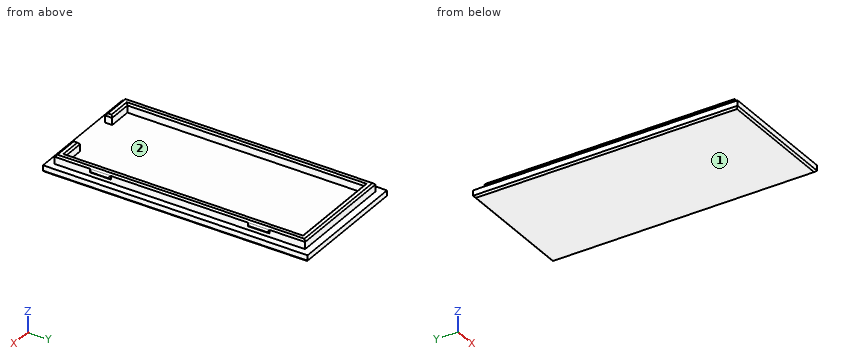
```python
from build123d import *

# Parameters (mm, degrees)
F1_W     = 2
F1_H     = 6.165323171
F1_H_2   = 5.8635988384
F1_H_3   = 38.7710779905
F1_W_2   = 14
F1_H_4   = 2
F1_W_3   = 26.8
F1_H_5   = 8
F1_W_4   = 0.5
F2_DEPTH = 2
F3_START = 1
F3_DEPTH = 3.5
F4_START = 3
F4_DEPTH = 1
F5_SIZE  = 0.49999


# Not quite as in the source:
# - a fillet or chamfer is up to 0.001 mm smaller than in the source, because OpenCascade refuses the exact size


with BuildPart() as f2:
    # F1 (on Top) → F2 (new body)
    with BuildSketch(Plane.XY):
        Polygon((16.0419130247, 37.7546238333), (-14.7580869753, 37.7546238333), (-14.7580869753, 27.7546238333), (-12.7580869753, 27.7546238333), (-12.7580869753, 35.7546238333), (14.0419130247, 35.7546238333), (14.0419130247, 27.7546238333), (16.0419130247, 27.7546238333), align=None)
        Polygon((-12.7580869753, -23.0453761667), (-14.7580869753, -23.0453761667), (-14.7580869753, -26.0453761667), (-14.7580869753, -33.0453761667), (-6.0801735182, -33.0453761667), (-6.0801735182, -31.0453761667), (-12.7580869753, -31.0453761667), align=None)
        with Locations((-13.7580869753, 24.6719622478)):
            Rectangle(F1_W, F1_H)
        with Locations((-13.7580869753, -20.1135767475)):
            Rectangle(F1_W, F1_H_2)
        Polygon((-12.7580869753, 21.5893006623), (-14.7580869753, 21.5893006623), (-14.7580869753, -3.2453761667), (-14.7580869753, -17.1817773283), (-12.7580869753, -17.1817773283), align=None)
        with Locations((15.0419130247, 2.203761667)):
            Rectangle(F1_W, F1_H_3)
        with Locations((15.0419130247, -20.1135767475)):
            Rectangle(F1_W, F1_H_2)
        Polygon((16.0419130247, -33.0453761667), (16.0419130247, -23.0453761667), (14.0419130247, -23.0453761667), (14.0419130247, -31.0453761667), (7.9198264818, -31.0453761667), (7.9198264818, -33.0453761667), align=None)
        with Locations((15.0419130247, 24.6719622478)):
            Rectangle(F1_W, F1_H)
        Polygon((-14.7580869753, -26.0453761667), (-16.7580869753, -26.0453761667), (-16.7580869753, -35.0453761667), (-6.0801735182, -35.0453761667), (-6.0801735182, -33.0453761667), (-14.7580869753, -33.0453761667), align=None)
        with Locations((0.9198264818, -32.0453761667)):
            Rectangle(F1_W_2, F1_H_4)
        with Locations((0.9198264818, -34.0453761667)):
            Rectangle(F1_W_2, F1_H_4)
        with Locations((0.6419130247, 24.6719622478)):
            Rectangle(F1_W_3, F1_H)
        with Locations((0.6419130247, 2.203761667)):
            Rectangle(F1_W_3, F1_H_3)
        Polygon((14.0419130247, -23.0453761667), (-12.7580869753, -23.0453761667), (-12.7580869753, -31.0453761667), (-6.0801735182, -31.0453761667), (7.9198264818, -31.0453761667), (14.0419130247, -31.0453761667), align=None)
        Polygon((-14.7580869753, 27.7546238333), (-14.7580869753, 37.7546238333), (16.0419130247, 37.7546238333), (16.0419130247, 27.7546238333), (16.5419130247, 27.7546238333), (16.5419130247, 21.5893006623), (16.0419130247, 21.5893006623), (16.0419130247, -17.1817773283), (16.5419130247, -17.1817773283), (16.5419130247, -23.0453761667), (16.0419130247, -23.0453761667), (16.0419130247, -33.0453761667), (7.9198264818, -33.0453761667), (7.9198264818, -35.0453761667), (18.0419130247, -35.0453761667), (18.0419130247, 39.7546238333), (-16.7580869753, 39.7546238333), (-16.7580869753, -3.2453761667), (-14.7580869753, -3.2453761667), (-14.7580869753, 21.5893006623), (-15.2580869753, 21.5893006623), (-15.2580869753, 27.7546238333), align=None)
        with Locations((0.6419130247, 31.7546238333)):
            Rectangle(F1_W_3, F1_H_5)
        Polygon((-14.7580869753, -17.1817773283), (-14.7580869753, -3.2453761667), (-16.7580869753, -3.2453761667), (-16.7580869753, -26.0453761667), (-14.7580869753, -26.0453761667), (-14.7580869753, -23.0453761667), (-15.2580869753, -23.0453761667), (-15.2580869753, -17.1817773283), align=None)
        with Locations((0.6419130247, -20.1135767475)):
            Rectangle(F1_W_3, F1_H_2)
        with Locations((-15.0080869753, -20.1135767475)):
            Rectangle(F1_W_4, F1_H_2)
        with Locations((-15.0080869753, 24.6719622478)):
            Rectangle(F1_W_4, F1_H)
        with Locations((16.2919130247, -20.1135767475)):
            Rectangle(F1_W_4, F1_H_2)
        with Locations((16.2919130247, 24.6719622478)):
            Rectangle(F1_W_4, F1_H)
    extrude(amount=F2_DEPTH)

    # F1 (on Top) → F3 (join)
    with BuildSketch(Plane.XY.offset(F3_START)):
        Polygon((16.0419130247, 37.7546238333), (-14.7580869753, 37.7546238333), (-14.7580869753, 27.7546238333), (-12.7580869753, 27.7546238333), (-12.7580869753, 35.7546238333), (14.0419130247, 35.7546238333), (14.0419130247, 27.7546238333), (16.0419130247, 27.7546238333), align=None)
        with Locations((-13.7580869753, 24.6719622478)):
            Rectangle(F1_W, F1_H)
        with Locations((15.0419130247, 24.6719622478)):
            Rectangle(F1_W, F1_H)
        with Locations((15.0419130247, 2.203761667)):
            Rectangle(F1_W, F1_H_3)
        Polygon((-12.7580869753, 21.5893006623), (-14.7580869753, 21.5893006623), (-14.7580869753, -3.2453761667), (-14.7580869753, -17.1817773283), (-12.7580869753, -17.1817773283), align=None)
        with Locations((15.0419130247, -20.1135767475)):
            Rectangle(F1_W, F1_H_2)
        Polygon((16.0419130247, -33.0453761667), (16.0419130247, -23.0453761667), (14.0419130247, -23.0453761667), (14.0419130247, -31.0453761667), (7.9198264818, -31.0453761667), (7.9198264818, -33.0453761667), align=None)
        Polygon((-12.7580869753, -23.0453761667), (-14.7580869753, -23.0453761667), (-14.7580869753, -26.0453761667), (-14.7580869753, -33.0453761667), (-6.0801735182, -33.0453761667), (-6.0801735182, -31.0453761667), (-12.7580869753, -31.0453761667), align=None)
        with Locations((-13.7580869753, -20.1135767475)):
            Rectangle(F1_W, F1_H_2)
    extrude(amount=F3_DEPTH)

    # F1 (on Top) → F4 (join)
    with BuildSketch(Plane.XY.offset(F4_START)):
        with Locations((-15.0080869753, 24.6719622478)):
            Rectangle(F1_W_4, F1_H)
        with Locations((-15.0080869753, -20.1135767475)):
            Rectangle(F1_W_4, F1_H_2)
        with Locations((16.2919130247, -20.1135767475)):
            Rectangle(F1_W_4, F1_H_2)
        with Locations((16.2919130247, 24.6719622478)):
            Rectangle(F1_W_4, F1_H)
    extrude(amount=F4_DEPTH)

    # F5 (size 0.5 in the source; OpenCascade refuses exactly that, so slightly less here)
    f5_edges = [f2.edges().sort_by_distance(p)[0] for p in [
        (0.641913, -35.045376, 0),
        (18.041913, 2.354624, 0),
        (0.641913, 39.754624, 0),
        (-16.758087, 2.354624, 0),
        (16.541913, -23.045376, 3.5),
        (16.541913, -17.181777, 3.5),
        (16.541913, -20.113577, 3),
        (16.541913, -20.113577, 4),
        (16.541913, 21.589301, 3.5),
        (16.541913, 27.754624, 3.5),
        (16.541913, 24.671962, 3),
        (16.541913, 24.671962, 4),
        (-15.258087, 27.754624, 3.5),
        (-15.258087, 21.589301, 3.5),
        (-15.258087, 24.671962, 3),
        (-15.258087, 24.671962, 4),
        (-15.258087, -17.181777, 3.5),
        (-15.258087, -23.045376, 3.5),
        (-15.258087, -20.113577, 3),
        (-15.258087, -20.113577, 4),
        (0.641913, 37.754624, 4.5),
        (-14.758087, 2.354624, 4.5),
        (-10.41913, -33.045376, 4.5),
        (-6.080174, -32.045376, 4.5),
        (-9.41913, -31.045376, 4.5),
        (-12.758087, 2.354624, 4.5),
        (0.641913, 35.754624, 4.5),
        (14.041913, 2.354624, 4.5),
        (10.98087, -31.045376, 4.5),
        (7.919826, -32.045376, 4.5),
        (11.98087, -33.045376, 4.5),
        (16.041913, 2.354624, 4.5),
    ]]
    chamfer(f5_edges, length=F5_SIZE)


solid = f2.part
```
CAD build for the part. Positions are in the model's coordinates, mm. Face numbers are marked on the shaded views. Coordinates: 2 decimals unless noted, no trailing zeros. Order: outer loops, then holes, each group sorted by start corner. A loop starts at its lowest first (then second) coordinate and runs counter-clockwise, first axis right, second up. Notation, with made-up numbers: (-12, 78.5) -> (24, 78.5) arc R30 ccw to (24, 115.5) -> close; hole circle Ø6 at (24.25, -27). An arc over 180 degrees is marked (long way). Use one line per item in the form item = value. Start each with the question number.
1) Pull direction Y, two halves, no side cores. Call the marked faces 1 and 2: +Y half, -Y half, draft (parallel to the pull), parting line (faces both ways), or undercut.
2) Band-saw the part on C-C on x = 11.5. Give the cut face in (y, z), then the cut area to 3 significant figures.
3) Band-saw the part on B-B on x = -3. Give the cut face in (y, z).
4) Drop flat-ended pins along their axis: pin 1 (2 mm diameter, centred on y = -3.5, z = 2.5, fed in from -X); pin 2 (0.6 mm diameter, centred on y = 19, z = 2.5, fed in from +X); pin 3 (1 mm diameter, centred on x = -3, y = -17, fed in from +Z); pin 4 (1.6 mm diameter, centred on y = -0.5, z = 3, fed in from -X). Give the stop position or say it passes through.
5) Drill centre lines: L1, parallel to X at y = 16.5, z = 3.8; L2, parallel to Y at x = -12.5, z = 2.9; L3, parallel to Z at x = 5, y = -28.5. Where is each one in solid material? Low to high. Write a range as [from, to].
6) Band-saw the part on A-A on y = -12. Give the cut face in (x, z), then the cut area to 4 significant figures.
Entries:
q1.face_1 = draft
q1.face_2 = undercut
q2.outline = (-35.05, 0.5) -> (-34.55, 0) -> (39.25, 0) -> (39.75, 0.5) -> (39.75, 2) -> (37.75, 2) -> (37.75, 4) -> (37.25, 4.5) -> (36.25, 4.5) -> (35.75, 4) -> (35.75, 2) -> (-31.05, 2) -> (-31.05, 4) -> (-31.55, 4.5) -> (-32.55, 4.5) -> (-33.05, 4) -> (-33.05, 2) -> (-35.05, 2) -> close
q2.area = 159 mm2
q3.outline = (-35.05, 0.5) -> (-34.55, 0) -> (39.25, 0) -> (39.75, 0.5) -> (39.75, 2) -> (37.75, 2) -> (37.75, 4) -> (37.25, 4.5) -> (36.25, 4.5) -> (35.75, 4) -> (35.75, 2) -> (-35.05, 2) -> close
q4.pin_1 = -16.76
q4.pin_2 = 16.04
q4.pin_3 = 2
q4.pin_4 = -14.76
q5.L1 = [-14.76, -12.76], [14.04, 16.04]
q5.L2 = [-33.05, -31.05], [35.75, 37.75]
q5.L3 = [0, 2]
q6.outline = (-16.76, 0.5) -> (-16.26, 0) -> (17.54, 0) -> (18.04, 0.5) -> (18.04, 2) -> (16.04, 2) -> (16.04, 4) -> (15.54, 4.5) -> (14.54, 4.5) -> (14.04, 4) -> (14.04, 2) -> (-12.76, 2) -> (-12.76, 4) -> (-13.26, 4.5) -> (-14.26, 4.5) -> (-14.76, 4) -> (-14.76, 2) -> (-16.76, 2) -> close
q6.area = 78.85 mm2
